Part model, mm, in its own coordinate system. A direction names the side the tool comes from. Give positions to 0.01 mm unless a question says otherwise; leave off trailing zeros. Use CSV: the item, a comma, the result in double quotes. Start each with the question number.
Item 1: Drill centre line: line 1 (X direction, y = 19, z = 16). Where is it in solid material? Low to high. Write a range as [from, to].
Item 2: Which spindle directions (+Z, -Z, +X, -X, +Y, -Y) get a long thin tool onto all of the face, cutting with end or side? Do faces 4 (the flat face through (39.09, 25, 12)), 5 (the flat face through (-68.562, -1, 12)). Say none if no direction does.
Item 3: Mould opens along X. For faces 1 (the flat face through (-1, -68.149, 12)), 2 (the flat face through (68.562, -1, 12)), 3 (the flat face through (-39.09, 25, 12)) say: released by +X, released by -X, zero draft, split by the parting line, or undercut.
from build123d import *

# Parameters (mm, degrees)
F0_W     = 137.1241360903
F0_H     = 136.2980902195
F1_DEPTH = 25


with BuildPart() as f1:
    # F0 (on Top) → F1 (new body)
    with BuildSketch(Plane.XY):
        Rectangle(F0_W, F0_H)
        with BuildLine():
            Line((-51.3400377035, 15.006557107), (-51.3400377035, 35.006557107))
            ThreePointArc((-51.3400377035, 35.006557107), (-51.2150377035, 35.131557107), (-51.0900377035, 35.006557107))
            Line((-51.0900377035, 35.006557107), (-51.0900377035, 15.006557107))
            ThreePointArc((-51.0900377035, 15.006557107), (-51.2150377035, 14.881557107), (-51.3400377035, 15.006557107))
        make_face(mode=Mode.SUBTRACT)
        with BuildLine():
            Line((-39.3400377035, 15.006557107), (-39.3400377035, 35.006557107))
            ThreePointArc((-39.3400377035, 35.006557107), (-39.2150377035, 35.131557107), (-39.0900377035, 35.006557107))
            Line((-39.0900377035, 35.006557107), (-39.0900377035, 15.006557107))
            ThreePointArc((-39.0900377035, 15.006557107), (-39.2150377035, 14.881557107), (-39.3400377035, 15.006557107))
        make_face(mode=Mode.SUBTRACT)
        with BuildLine():
            ThreePointArc((39.0900377035, 35.006557107), (39.2150377035, 35.131557107), (39.3400377035, 35.006557107))
            Line((39.3400377035, 35.006557107), (39.3400377035, 15.006557107))
            ThreePointArc((39.3400377035, 15.006557107), (39.2150377035, 14.881557107), (39.0900377035, 15.006557107))
            Line((39.0900377035, 15.006557107), (39.0900377035, 35.006557107))
        make_face(mode=Mode.SUBTRACT)
        with BuildLine():
            ThreePointArc((51.3400377035, 15.006557107), (51.2150377035, 14.881557107), (51.0900377035, 15.006557107))
            Line((51.0900377035, 15.006557107), (51.0900377035, 35.006557107))
            ThreePointArc((51.0900377035, 35.006557107), (51.2150377035, 35.131557107), (51.3400377035, 35.006557107))
            Line((51.3400377035, 35.006557107), (51.3400377035, 15.006557107))
        make_face(mode=Mode.SUBTRACT)
    extrude(amount=F1_DEPTH)


solid = f1.part
Worked answers:
1,line 1,"x = [-68.56, -51.34], [-51.09, -39.34], [-39.09, 39.09], [39.34, 51.09], [51.34, 68.56]"
2,face 4,"+Z, -Z"
2,face 5,"+Z, -Z, -X, +Y, -Y"
3,face 1,"zero draft"
3,face 2,"released by +X"
3,face 3,"undercut"
